Autodesk Fusion 360 part; units mm, degrees
sketch "Sketch1" plane through (0, 0, 0) normal (0, 0, 1) x (1, 0, 0)
  circle A0 centre (0, 0) radius 4
  line L0 (0, -7.5056) -> (6.5, -3.7528)
  line L1 (6.5, -3.7528) -> (6.5, 3.7528)
  line L2 (6.5, 3.7528) -> (0, 7.5056)
  line L3 (0, 7.5056) -> (-6.5, 3.7528)
  line L4 (-6.5, 3.7528) -> (-6.5, -3.7528)
  line L5 (-6.5, -3.7528) -> (0, -7.5056)
  dimension "d1" = 8
  dimension "d2" = 13
extrude "Extrude1" add sketch "Sketch1" along normal blind 3.5
fillet "Fillet1" radius 0.5 20 edges at (-3.7293, 1.4465, 0) (-6.5, -3.7528, 1.75) (3.25, 5.6292, 0) (-3.25, 5.6292, 3.5) (3.25, -5.6292, 3.5) (6.5, 3.7528, 1.75) (6.5, 0, 0) (-6.5, 0, 0) (-6.5, 3.7528, 1.75) (6.5, -3.7528, 1.75) (-3.25, -5.6292, 3.5) (-6.5, 0, 3.5) (3.25, -5.6292, 0) (-3.25, -5.6292, 0) (-3.7293, 1.4465, 3.5) (0, 7.5056, 1.75) (0, -7.5056, 1.75) (3.25, 5.6292, 3.5) (6.5, 0, 3.5) (-3.25, 5.6292, 0) 9 faces at (-6.5, 1.2509, 1.1667) (6.5, -1.2509, 1.1667) (-2.1667, 6.2546, 1.1667) (2.1667, -6.2546, 1.1667) (3.9801, -0.3983, 2.3333) (-4.3333, -5.0037, 1.1667) (5.6667, 0, 3.5) (5.6667, 0, 0) (4.3333, 5.0037, 1.1667)
Can you work these out from the model? Positions are in its coordinate system, mm. Give positions to 0.01 mm unless a question says otherwise; leave off trailing zeros. Order: outer loops, then holes, each group sorted by start corner. A loop starts at its lowest first (then second) coordinate and runs counter-clockwise, first axis right, second up. Notation, with made-up numbers: M -25,19.5 L -6,19.5 A29 ccw -6,58.5 Z; hole C 11.5,-5.75 d11. An arc over 180 degrees is marked long. Write item = value, one per line. Start each with the question number.
Q1. I need wall thicknesses on probe 1 along Y at (x, z) = (0, 1.85); probe 2 along X at (y, z) = (-1.25, 2.45); probe 3 along X at (y, z) = (-0.75, 1.6). Which ranges of each line are inside material? Lowest first, please. Write a range as [from, to].
Q2. Suppose I cut it at A-A (y = 0). Write out the boundary of the cut face in (x, z).
Q3. Suppose I cut it at B-B (z = 2.25). Write out the boundary of the cut face in (x, y).
Q4. Suppose I cut it at C-C (z = 3.2). Write out the boundary of the cut face in (x, y), plus the area to 3 significant figures.
Q5. We'd pull the mould along X, two halves only. Please class faces 1 (the flat face through (-3.21, 5.65, 1.73)), 2 (the cylindrical face through (-0.867, 3.905, 1.732)), 3 (the flat face through (3.21, -5.65, 1.73)), 4 (the flat face through (0, -5, 3.5)): pulls with the +X half, pulls with the -X half, needs draft (parallel to the pull), parting line crosses it, or undercut.
Q6. Will these pins go through, and if not, where does the flat tip stop? pin 1 Ø5 at (x, y) = (0, 0) entering from +Z; pin 2 Ø1 at (x, z) = (5, 3) entering from -Y.
Check result:
q1.probe_1 = [-7.43, -4], [4, 7.43]
q1.probe_2 = [-6.5, -3.8], [3.8, 6.5]
q1.probe_3 = [-6.5, -3.93], [3.93, 6.5]
q2.outline = M -6.5,0.5 A0.5 ccw -6,0 L -4.5,0 A0.5 ccw -4,0.5 L -4,3 A0.5 ccw -4.5,3.5 L -6,3.5 A0.5 ccw -6.5,3 Z; M 4,0.5 A0.5 ccw 4.5,0 L 6,0 A0.5 ccw 6.5,0.5 L 6.5,3 A0.5 ccw 6,3.5 L 4.5,3.5 A0.5 ccw 4,3 Z
q3.outline = M -6.5,-3.46 A0.5 ccw -6.25,-3.9 L -0.25,-7.36 A0.5 ccw 0.25,-7.36 L 6.25,-3.9 A0.5 ccw 6.5,-3.46 L 6.5,3.46 A0.5 ccw 6.25,3.9 L 0.25,7.36 A0.5 ccw -0.25,7.36 L -6.25,3.9 A0.5 ccw -6.5,3.46 Z; hole C 0,0 d8
q4.outline = M -6.46,-3.46 A0.46 ccw -6.23,-3.86 L -0.23,-7.33 A0.46 ccw 0.23,-7.33 L 6.23,-3.86 A0.46 ccw 6.46,-3.46 L 6.46,3.46 A0.46 ccw 6.23,3.86 L 0.23,7.33 A0.46 ccw -0.23,7.33 L -6.23,3.86 A0.46 ccw -6.46,3.46 Z; hole C 0,0 d8.08
q4.area = 93.1 mm2
q5.face_1 = pulls with the -X half
q5.face_2 = undercut
q5.face_3 = pulls with the +X half
q5.face_4 = needs draft
q6.pin_1 = through
q6.pin_2 = -4.91
